from build123d import *

# Parameters (mm, degrees)
SKETCH2_R             = 12.7
SKETCH2_R_2           = 3.175
BOSS_EXTRUDE1_DEPTH   = 3.175
CHAMFER1_SIZE         = 0.254
F_6_32_TAPPED_HOLE1_D = 2.7051


# Read off the part's stored shape, not the designer's step: #4-40 Tapped Hole2
with BuildPart() as part:
    # Sketch2 → Boss-Extrude1 (new, symmetric)
    with BuildSketch(Plane.XY):
        Circle(SKETCH2_R)
        Circle(SKETCH2_R_2, mode=Mode.SUBTRACT)
    extrude(amount=BOSS_EXTRUDE1_DEPTH, both=True)

    # Chamfer1
    chamfer1_edges = [part.edges().sort_by_distance(p)[0] for p in [
        (-12.7, 0, -3.175),
        (-12.7, 0, 3.175),
    ]]
    chamfer(chamfer1_edges, length=CHAMFER1_SIZE)

    # #6-32 Tapped Hole1 (through all)
    with Locations(Plane.XY.offset(3.175)):
        with Locations((0, 7.9502), (6.885075165, -3.9751), (-6.885075165, -3.9751)):
            Hole(F_6_32_TAPPED_HOLE1_D / 2)

    # #4-40 Tapped Hole2 outline → #4-40 Tapped Hole2 (revolve, cut)
    with BuildSketch(Plane.XY):
        Polygon((0, -12.700018831), (1.473216369, -12.700018831), (1.1303, -12.305538673), (1.1303, -2.966966147), (0, -2.966966147), align=None)
    revolve(axis=Axis((0, 0, 0), (0, 1, 0)), mode=Mode.SUBTRACT)


solid = part.part
Part model, mm, in its own coordinate system. Coordinates: 2 decimals unless noted, no trailing zeros. Write each loop counter-clockwise with the first axis right and the second up, starting at its lowest first coordinate (ties: lowest second). Pieces come first, ordered by that corner, then holes. Notation, with made-up numbers: (74, 36.5) - (131, 36.5) arc R20 cw to (131, 61.5) - close; hole circle Ø2 at (80.5, 68). An arc over 180 degrees is marked (long way). Put each result on its own line as item: value.
1. Band-saw the part on B-B (x = 0). Write the cut outline in (y, z) (3 decimals).
Final values:
outline: (-12.7, -2.921) - (-12.446, -3.175) - (-3.175, -3.175) - (-3.175, -1.13) - (-12.306, -1.13) - (-12.7, -1.473) - close; (-12.7, 1.473) - (-12.306, 1.13) - (-3.175, 1.13) - (-3.175, 3.175) - (-12.446, 3.175) - (-12.7, 2.921) - close; (3.175, -3.175) - (6.598, -3.175) - (6.598, 3.175) - (3.175, 3.175) - close; (9.303, -3.175) - (12.446, -3.175) - (12.7, -2.921) - (12.7, 2.921) - (12.446, 3.175) - (9.303, 3.175) - close
2. Band-saw the part on A-A (y = 0). Write the cut outline in (x, z) (3 decimals).
Final values:
outline: (-12.7, -2.921) - (-12.446, -3.175) - (-3.175, -3.175) - (-3.175, 3.175) - (-12.446, 3.175) - (-12.7, 2.921) - close; (3.175, -3.175) - (12.446, -3.175) - (12.7, -2.921) - (12.7, 2.921) - (12.446, 3.175) - (3.175, 3.175) - close
3. Band-saw the part on C-C (z = 2). Write the cut outline in (x, y) (3 decimals), then the cut area to 3 significant figures.
Final values:
outline: circle Ø25.4 at (0, 0); hole circle Ø2.705 at (-6.885, -3.975); hole circle Ø6.35 at (0, 0); hole circle Ø2.705 at (0, 7.95); hole circle Ø2.705 at (6.885, -3.975)
area: 458 mm²
4. Flat gauge pins, fed straight in: pin 1 Ø1 at (y, z) = (2.5, -0.5) entering from +X; pin 2 Ø3 at (x, z) = (-7.5, 2) entering from +Y; pin 3 Ø1 at (x, z) = (-2, 1.5) entering from +Y. Where does each tip first touch, or does it go through?
Final values:
pin 1: stops at x = 12.54
pin 2: stops at y = 11.19
pin 3: stops at y = 12.61
5. Two-plate mould, pull along Z, no slides. Class faces 1 (the cylindrical face through (-0.245, -7.571, 1.103)), 2 (the flat face through (3, -3, -3.175)), 3 (the cylindrical face through (-8.175, -3.569, -0.044)): +Z half, -Z half, draft (parallel to the pull), parting line (faces both ways), or undercut.
Final values:
face 1: undercut
face 2: -Z half
face 3: draft
6. Band-saw the part on D-D (z = 0). Write the cut outline in (x, y) (3 decimals).
Final values:
outline: (-1.405, -12.622) - (-1.13, -12.306) - (-1.13, -2.967) arc R3.175 cw (long way) to (1.13, -2.967) - (1.13, -12.306) - (1.405, -12.622) arc R12.7 ccw (long way) to start; hole circle Ø2.705 at (-6.885, -3.975); hole circle Ø2.705 at (0, 7.95); hole circle Ø2.705 at (6.885, -3.975)
7. Probe line 1 along Y through (x, z) = (0, 1.25) (3 decimals); line 2 along Z through (x, y) = (0, -8.25) (3 decimals); line 3 along Y through (x, z) = (0, 2) (3 decimals). List the from-to ranges inside material, lowest first. Write a range as [from, to].
Final values:
line 1: y = [-12.443, -3.175], [3.175, 6.598], [9.303, 12.7]
line 2: z = [-3.175, -1.13], [1.13, 3.175]
line 3: y = [-12.7, -3.175], [3.175, 6.598], [9.303, 12.7]
